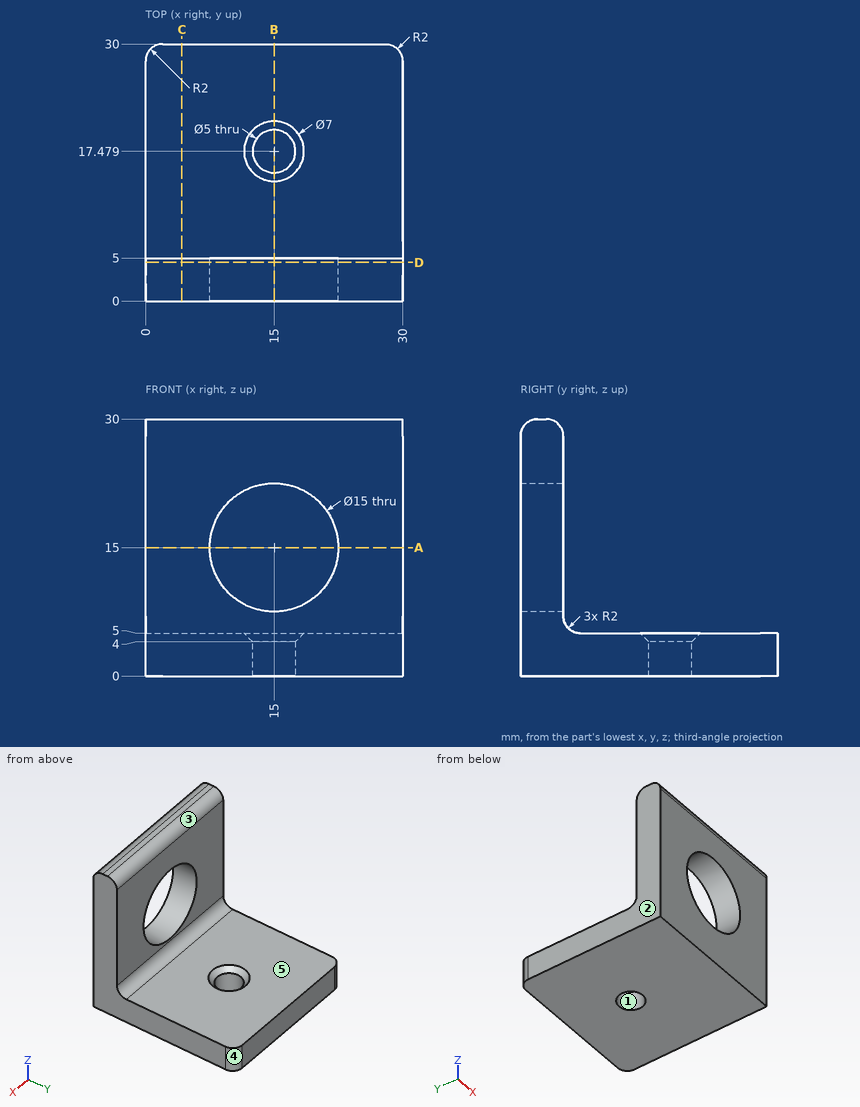
Answer from the drawing. Dimensions are ordinates in mm from the lowest x, y and z of the part. A direction names the side the tool comes from. Give positions to 0.01 mm unless a question says otherwise; leave off trailing zeros. Write each loop counter-clockwise with the first axis right and the second up, starting at its lowest first coordinate (ties: lowest second). Pieces come first, ordered by that corner, then holes. Notation, with made-up numbers: M 48.5,-31 L 99.5,-31 A14 cw 99.5,-27 Z; hole C 36.5,51 d10. An arc over 180 degrees is marked long. Answer as CSV lines item,"result".
Q1. A cutting plane is placed at A-A on z = 15. Write down the section's boundary in (x, y), plus the area to 3 significant figures.
A:
outline,"M 0,0 L 7.5,0 L 7.5,5 L 0,5 Z; M 22.5,0 L 30,0 L 30,5 L 22.5,5 Z"
area,"75.0 mm²"
Q2. The mould has two halves that part along Y. Classify the marked faces 1, 2 and 3: +Y half, -Y half, draft (parallel to the pull), parting line (faces both ways), or undercut.
A:
face 1,"undercut"
face 2,"draft"
face 3,"+Y half"
Q3. A cutting plane is placed at B-B on x = 15. Write down the section's boundary in (y, z), plus the area to 3 significant figures.
A:
outline,"M 0,0 L 14.98,0 L 14.98,4 L 13.98,5 L 7,5 A2 cw 5,7 L 5,7.5 L 0,7.5 Z; M 0,22.5 L 5,22.5 L 5,28 A2 ccw 3,30 L 2,30 A2 ccw 0,28 Z; M 19.98,0 L 30,0 L 30,5 L 20.98,5 L 19.98,4 Z"
area,"173 mm²"
Q4. A cutting plane is placed at C-C on x = 4.25. Write down the section's boundary in (y, z).
A:
outline,"M 0,0 L 30,0 L 30,5 L 7,5 A2 cw 5,7 L 5,28 A2 ccw 3,30 L 2,30 A2 ccw 0,28 Z"
Q5. A cutting plane is placed at D-D on y = 4.5. Write down the section's boundary in (x, z), plus the area to 3 significant figures.
A:
outline,"M 0,0 L 30,0 L 30,29.32 L 0,29.32 Z; hole C 15,15 d15"
area,"703 mm²"
Q6. A tool of negligible diameter and unlimited length cuts with its end or side. For the marked faces 4 and 5, from which of +Z, -Z, +X, -X, +Y, -Y can it reach the whole face along a straight path? Write none if from no direction.
A:
face 4,"+Z, -Z, +X, +Y"
face 5,"+Z, +X, -X, +Y"
Q7. Given P1, Ø3, axis at x = 18, y = 19.5, coming from the +Z side; P2, Ø4, axis at x = 18.5, y = 5.5, coming from the +Z side, each flat-ended and moving along its own axis, determine where each tip first touches the part or whether it passes through.
A:
P1,"stops at z = 5"
P2,"stops at z = 29.94"
Q8. Find the intervals of material crossed by probe 1 along X at (y, z) = (1.4, 15); probe 2 along Z at (x, y) = (6.75, 17), in increasing order. Write a range as [from, to].
A:
probe 1,"x = [0, 7.5], [22.5, 30]"
probe 2,"z = [0, 5]"
